Can you work these out from the drawing? Everything is in mm from the part's minimum corner. A direction names the side the tool comes from. Give positions to 0.01 mm unless a question says otherwise; leave off trailing zeros. Order: outer loops, then holes, each group sorted by start corner. A loop starts at its lowest first (then second) coordinate and runs counter-clockwise, first axis right, second up. Notation, with made-up numbers: (-10, 25) -> (42, 25) arc R9 cw to (42, 33) -> close; hole circle Ø8 at (18, 67). An arc over 180 degrees is marked (long way). Answer as CSV lines item,"result". Start each with the question number.
(1) I want a section at D-D (y = 103). Please give me the cut outline in (x, z), plus the area to 3 significant figures.
(2) I want a section at B-B (x = 23). Please give me the cut outline in (y, z).
(3) I want a section at A-A (y = 127.5). Please give me the cut outline in (x, z).
(4) I need wall thicknesses on L1, parallel to X at y = 176.5, z = 93; L2, parallel to Y at x = 101, z = 55. Which ranges of each line are inside material? Lowest first, please.
(5) Will these pins go through, and if not, where does the flat tip stop? pin 1 Ø6 at (y, z) = (40.5, 53) entering from -X; pin 2 Ø10 at (x, z) = (47.5, 39) entering from +Y; pin 3 Ø6 at (x, y) = (80, 26) entering from +Z; pin 4 Ø10 at (x, z) = (62.5, 92) entering from -Y.
(6) I want a section at C-C (z = 55). Please give me the cut outline in (x, y), plus the area to 3 significant figures.
(7) On a 3-axis mill with a long thin cutter (end or side, diameter ignored), from which of +Z, -Z, +X, -X, +Y, -Y can I reach the whole of each face in a straight line? I mean the marked faces 4, 5 and 6. Say none if no direction works.
(8) We'd pull the mould along Z, two halves only. Please class the marked faces 1, 2 and 3: released by +Z, released by -Z, zero draft, split by the parting line, or undercut.
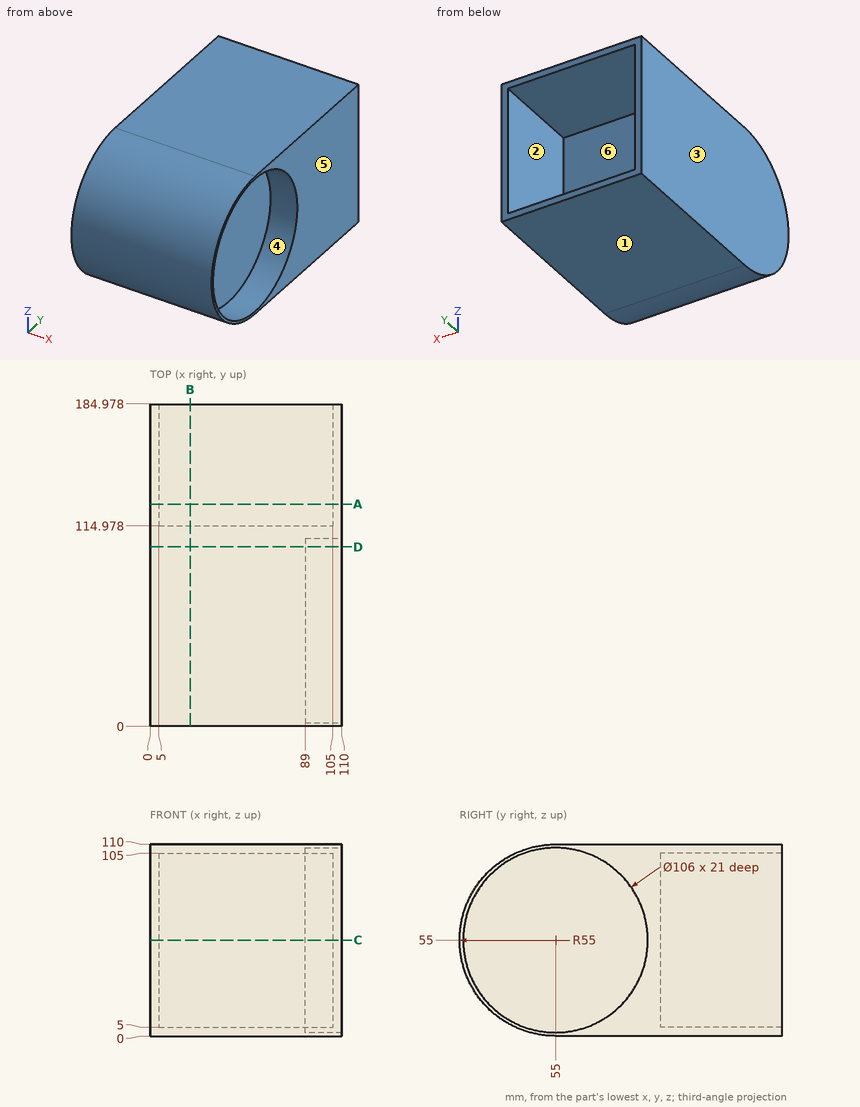
Final values:
1,outline,"(0, 0) -> (110, 0) -> (110, 32.53) -> (89, 32.53) -> (89, 77.47) -> (110, 77.47) -> (110, 110) -> (0, 110) -> close"
1,area,"11,200 mm²"
2,outline,"(55, 0) -> (184.98, 0) -> (184.98, 5) -> (114.98, 5) -> (114.98, 105) -> (184.98, 105) -> (184.98, 110) -> (55, 110) arc R55 ccw to start"
3,outline,"(0, 0) -> (110, 0) -> (110, 110) -> (0, 110) -> close; hole (5, 5) -> (105, 5) -> (105, 105) -> (5, 105) -> close"
4,L1,"0 to 5, 105 to 110"
4,L2,"0 to 2, 108 to 114.98"
5,pin 1,"x = 0"
5,pin 2,"y = 114.98"
5,pin 3,"z = 103.47"
5,pin 4,"y = 10.27"
6,outline,"(0, 0) -> (110, 0) -> (110, 2) -> (89, 2) -> (89, 108) -> (110, 108) -> (110, 184.98) -> (105, 184.98) -> (105, 114.98) -> (5, 114.98) -> (5, 184.98) -> (0, 184.98) -> close"
6,area,"11,100 mm²"
7,face 4,"+X"
7,face 5,"+Z, -Z, +X, +Y, -Y"
7,face 6,"+Y"
8,face 1,"released by -Z"
8,face 2,"undercut"
8,face 3,"zero draft"
